Check sheet for the modelled part. Datum: model origin and axes. Units: mm. A direction names the side the tool comes from. Round coordinates to 2 decimals unless told otherwise and drop trailing zeros. Order: outer loops, then holes, each group sorted by start corner. A loop starts at its lowest first (then second) coordinate and runs counter-clockwise, first axis right, second up.
Q1. Set-up check for faces 1 (the flat face through (3.2, 2, 4)), 2 (the flat face through (0, 2, 2)): record each of +Z, -Z, +X, -X, +Y, -Y from which the full face is reachable in a straight line by a thin tool's end or side.
Q2. Scan lines: probe 1 along Z at (x, y) = (3.9, 2.5); probe 2 along Z at (x, y) = (2.65, 2.5); probe 3 along Z at (x, y) = (4.35, 1.3). Record each from-to range of solid material in increasing order.
Q3. Cross-section at D-D on x = 4.4. Record the cut outline in (y, z).
Q4. Cross-section at B-B on x = 2. Record the cut outline in (y, z), then the cut area to 3 significant figures.
Q5. Cross-section at C-C on y = 2.35. Record the cut outline in (x, z), then the cut area to 3 significant figures.
Q6. Depth check by flat-ended pin: P1, Ø1, axis at x = 3.5, z = 1.5, coming from the -Y side. Enter the tip coordinate at first touch or a pass-through.
Q7. Cross-section at A-A on z = 2. Record the cut outline in (x, y).
from build123d import *

# Parameters (mm, degrees)
F1_DEPTH = 4
F3_DEPTH = 1
F4_R     = 0.5
F5_DEPTH = 4
F6_R     = 0.25
F7_DEPTH = 25


with BuildPart() as f1:
    # F0 (on Top) → F1 (new body)
    with BuildSketch(Plane.XY):
        Polygon((0, 2), (0, 0), (5, 0), (5, 4), (2, 4), (0, 4), align=None)
    extrude(amount=F1_DEPTH)

    # F2 (on face) → F3 (join)
    with BuildSketch(Plane.XY.offset(4)):
        with BuildLine():
            ThreePointArc((1, 2), (2, 1), (3, 2))
            ThreePointArc((3, 2), (2, 3), (1, 2))
        make_face()
    extrude(amount=F3_DEPTH)

    # F4 (on face) → F5 (cut)
    with BuildSketch(Plane(origin=(0, 4, 0), x_dir=(-1, 0, 0), z_dir=(0, 1, 0))):
        with Locations((-5, 4)):
            Circle(F4_R)
    extrude(amount=-F5_DEPTH, mode=Mode.SUBTRACT)

    # F6 (on face) → F7 (cut)
    with BuildSketch(Plane.YZ.offset(5)):
        with Locations((2.5, 2)):
            Circle(F6_R)
    extrude(amount=-F7_DEPTH, mode=Mode.SUBTRACT)


solid = f1.part
Results found:
1. face 1: +Z
1. face 2: +Z, -Z, -X, +Y, -Y
2. probe 1: z = 0 to 1.75, 2.25 to 4
2. probe 2: z = 0 to 1.75, 2.25 to 5
2. probe 3: z = 0 to 4
3. outline: (0, 0) - (4, 0) - (4, 4) - (0, 4) - close; hole circle Ø0.5 at (2.5, 2)
4. outline: (0, 0) - (4, 0) - (4, 4) - (3, 4) - (3, 5) - (1, 5) - (1, 4) - (0, 4) - close; hole circle Ø0.5 at (2.5, 2)
4. area: 17.8 mm2
5. outline: (0, 0) - (5, 0) - (5, 1.8) - (0, 1.8) - close; (0, 2.2) - (5, 2.2) - (5, 3.5) arc R0.5 cw to (4.5, 4) - (2.94, 4) - (2.94, 5) - (1.06, 5) - (1.06, 4) - (0, 4) - close
5. area: 19.7 mm2
6. P1: stops at y = 0
7. outline: (0, 0) - (5, 0) - (5, 2.25) - (0, 2.25) - close; (0, 2.75) - (5, 2.75) - (5, 4) - (0, 4) - close
